Check sheet for the drawn part. Datum: minimum x, y, z corner. Units: mm. A direction names the side the tool comes from. Give positions to 0.01 mm unless a question says otherwise; leave off trailing zeros. Write each loop counter-clockwise with the first axis right and the second up, starting at its lowest first coordinate (ties: lowest second). Pieces come first, ordered by that corner, then holes.
(1) Tool access check on the marked faces 4 and 5. Record the directions out of +Z, -Z, +X, -X, +Y, -Y that give a thin tool (end or side, any length) a straight path to the whole face; none if there is none.
(2) Cross-section at C-C (x = 34). Record the boundary of the cut face in (y, z).
(3) Cross-section at D-D (x = 48). Record the boundary of the cut face in (y, z), and give its area (3 significant figures).
(4) Cross-section at B-B (z = 75.5). Record the boundary of the cut face in (x, y), and give its area (3 significant figures).
(5) Thickness scan on line 1 along X through (y, z) = (12.5, 31); line 2 along Z through (x, y) = (27, 17.5); line 3 along Z through (x, y) = (50, 6.75). Record the ranges inside material, lowest first.
(6) Depth check by flat-ended pin: P1, Ø4, axis at x = 31, y = 13, coming from the -Z side; P2, Ø6, axis at x = 50.5, y = 14.5, coming from the -Z side; P3, Ø3, axis at x = 47.5, y = 3.5, coming from the -Z side; P4, Ø6, axis at y = 7, z = 86, coming from the -X side. Enter the tip coordinate at first touch or a pass-through.
(7) Cross-section at A-A (y = 16.25). Record the boundary of the cut face in (x, z).
(8) Mould release check, pull along X, two halves, no side actions. Record for the marked faces 1, 2 and 3: +X half, -X half, draft (parallel to the pull), parting line (faces both ways), or undercut.
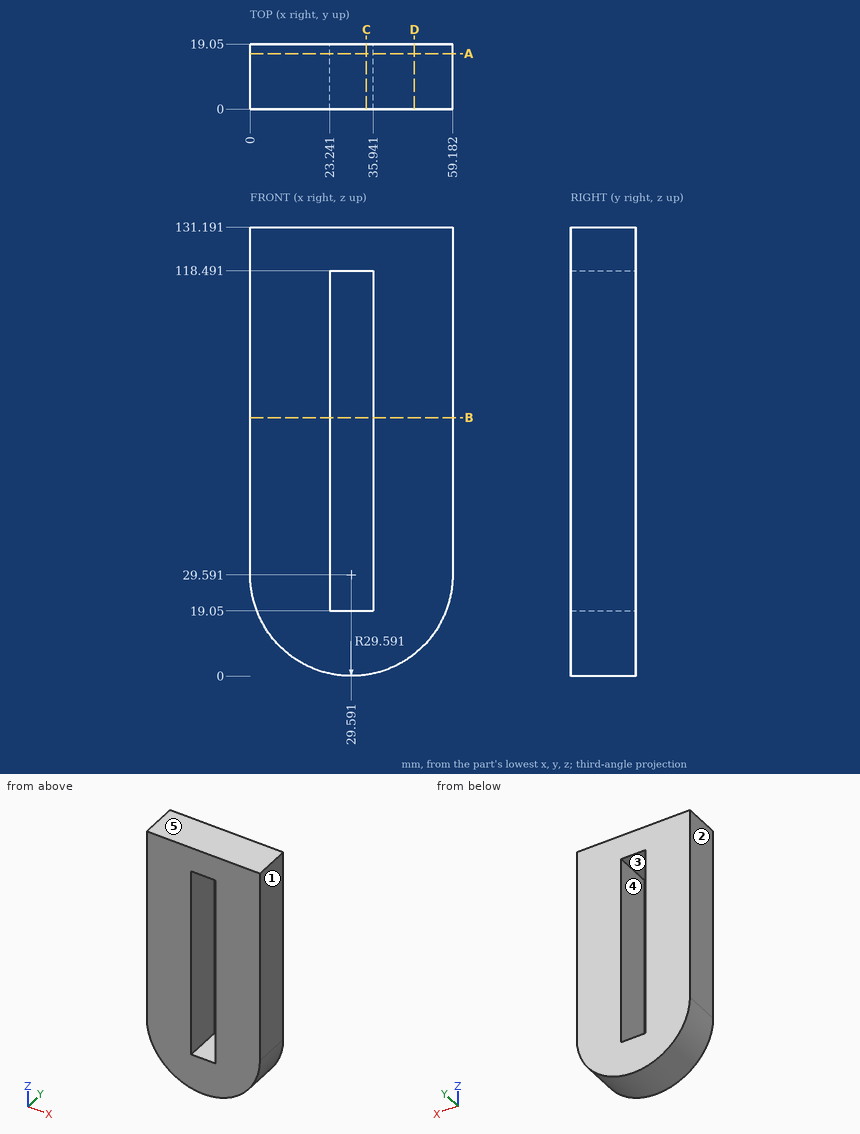
Reply:
1. face 4: +Y, -Y
1. face 5: +Z, +X, -X, +Y, -Y
2. outline: (0, 0.33) - (19.05, 0.33) - (19.05, 19.05) - (0, 19.05) - close; (0, 118.49) - (19.05, 118.49) - (19.05, 131.19) - (0, 131.19) - close
3. outline: (0, 6.42) - (19.05, 6.42) - (19.05, 131.19) - (0, 131.19) - close
3. area: 2,380 mm2
4. outline: (0, 0) - (23.24, 0) - (23.24, 19.05) - (0, 19.05) - close; (35.94, 0) - (59.18, 0) - (59.18, 19.05) - (35.94, 19.05) - close
4. area: 885 mm2
5. line 1: x = 0 to 23.24, 35.94 to 59.18
5. line 2: z = 0.11 to 19.05, 118.49 to 131.19
5. line 3: z = 8.16 to 131.19
6. P1: stops at z = 0
6. P2: stops at z = 6.03
6. P3: stops at z = 4.97
6. P4: stops at x = 0
7. outline: (0, 29.59) arc R29.59 ccw to (59.18, 29.59) - (59.18, 131.19) - (0, 131.19) - close; hole (23.24, 19.05) - (35.94, 19.05) - (35.94, 118.49) - (23.24, 118.49) - close
8. face 1: +X half
8. face 2: -X half
8. face 3: undercut
